```python
from build123d import *

# Parameters (mm, degrees)
CYLINDER009_R     = 2.65
CYLINDER009_DEPTH = 30
CYLINDER008_R     = 4
CYLINDER008_DEPTH = 3.2
CYLINDER010_R     = 1.375
CYLINDER010_DEPTH = 10
CYLINDER011_R     = 2.6
CYLINDER011_DEPTH = 2.1
ARRAY002_X_COUNT  = 2
ARRAY002_X_PITCH  = 15
CYLINDER007_R     = 37.7
CYLINDER007_DEPTH = 63


with BuildPart() as cylinder009:
    # Cylinder009 → Cylinder009 (new body)
    with BuildSketch(Plane.XY.offset(63)):
        Circle(CYLINDER009_R)
    extrude(amount=CYLINDER009_DEPTH)


with BuildPart() as cylinder008:
    # Cylinder008 → Cylinder008 (new body)
    with BuildSketch(Plane.XY.offset(64.8)):
        Circle(CYLINDER008_R)
    extrude(amount=CYLINDER008_DEPTH)


with BuildPart() as cylinder010:
    # Cylinder010 → Cylinder010 (new body)
    with BuildSketch(Plane.XY):
        Circle(CYLINDER010_R)
    extrude(amount=CYLINDER010_DEPTH)


with BuildPart() as fusion005:
    # Cylinder011 → Cylinder011 (new body)
    with BuildSketch(Plane.XY):
        Circle(CYLINDER011_R)
    extrude(amount=CYLINDER011_DEPTH)

    # Fusion004: union Cylinder010
    add(cylinder010.part)


with BuildPart() as fusion005_1:
    # Fusion004 placement: moved
    add(fusion005.part.moved(Location((0, 0, 63))))

    # Array002 X: Fusion005 ×2


with BuildPart() as fusion005_2:
    add(fusion005_1.part)
    with Locations(*[(i * ARRAY002_X_PITCH, 0, 0) for i in range(1, ARRAY002_X_COUNT)]):
        add(fusion005_1.part)


with BuildPart() as fusion005_3:
    # Array002 placement: moved
    add(fusion005_2.part.moved(Location((-7.5, 0, 0))))

    # Fusion005: union Cylinder009, Cylinder008
    add(cylinder009.part)
    add(cylinder008.part)


with BuildPart() as cut007:
    # Cylinder007 → Cylinder007 (new body)
    with BuildSketch(Plane.XY):
        Circle(CYLINDER007_R)
    extrude(amount=CYLINDER007_DEPTH)

    # Cut007: cut Fusion005
    add(fusion005_3.part, mode=Mode.SUBTRACT)


solid = cut007.part
```
The listing builds one solid part. Answer for the finished solid, in the listing's coordinates (mm). Round coordinates to 2 decimals unless told otherwise and drop trailing zeros. Loops run counter-clockwise (first coordinate to the right, second up) from the corner with the lowest first, then second, coordinate; pieces in that order, holes last. Notation, with made-up numbers: (4.5, 49.5) - (22.5, 49.5) arc R16 cw to (22.5, 55.5) - close; hole circle Ø8 at (-37.75, 89.5). An arc over 180 degrees is marked (long way). Use one line per item in the form item = value. Start each with the question number.
1. The part is cut by section B-B on x = 13.5. Determine the outline of the cut face in (y, z), then the cut area to 3 significant figures.
2. The part is cut by section A-A on z = 28.5. Determine the outline of the cut face in (x, y).
3. The part is cut by section C-C on y = 22. Determine the outline of the cut face in (x, z).
4. Consider line 1 (Y direction, x = 31.5, z = 60); line 2 (X direction, y = -5, z = 43); line 3 (X direction, y = -8, z = 49). Determine where each line is inside the solid, lowest interval first. Write a range as [from, to].
5. Given pin 1 Ø2 at (x, z) = (-28, 49.5) entering from +Y; pin 2 Ø1 at (y, z) = (-29.5, 8) entering from -X; pin 3 Ø2 at (x, z) = (0, 28) entering from -Y, each flat-ended and moving along its own axis, determine where each tip first touches the part or whether it passes through.
Geometry check:
q1.outline = (-35.2, 0) - (35.2, 0) - (35.2, 63) - (-35.2, 63) - close
q1.area = 4,440 mm^2
q2.outline = circle Ø75.4 at (0, 0)
q3.outline = (-30.62, 0) - (30.62, 0) - (30.62, 63) - (-30.62, 63) - close
q4.line_1 = [-20.71, 20.71]
q4.line_2 = [-37.37, 37.37]
q4.line_3 = [-36.84, 36.84]
q5.pin_1 = 26.31
q5.pin_2 = -24.09
q5.pin_3 = -37.7
